The drawing under review shows one solid part. Ordinate dimensions are in mm from its lowest x, y, z. A direction names the side the tool comes from. Coordinates: 2 decimals unless noted, no trailing zeros. Write each loop counter-clockwise with the first axis right and the second up, starting at its lowest first coordinate (ties: lowest second). Pieces come first, ordered by that corner, then holes. Notation, with made-up numbers: (36.25, 67) -> (92.25, 67) arc R24 cw to (92.25, 84) -> close; hole circle Ø4 at (35.25, 63). An arc over 180 degrees is marked (long way). One line per item, written item: value. Start each with the question number.
1) For pin 1 Ø5 at (x, y) = (132, 98.5) entering from +Z, flat-tipped, find the tip position at first contact; note if it passes through.
2) Add section B-B (y = 104.5). State the section outline as (x, z) points, and give its area (3 significant figures).
3) Add section A-A (x = 173.5). State the section outline as (y, z) points, and give its area (3 significant figures).
4) For probe 1 along Z at (x, y) = (302.5, 147.5); probe 2 along Y at (x, z) = (127, 7.25), list the stretches that pass through material, from the lowest coordinate up. Write a range as from..to.
5) Machinability: for the marked faces 1 and 2, which of the approach directions +Z, -Z, +X, -X, +Y, -Y give a long, thin tool a straight path to every point of the face, cutting with its end or side? Answer none if there is none.
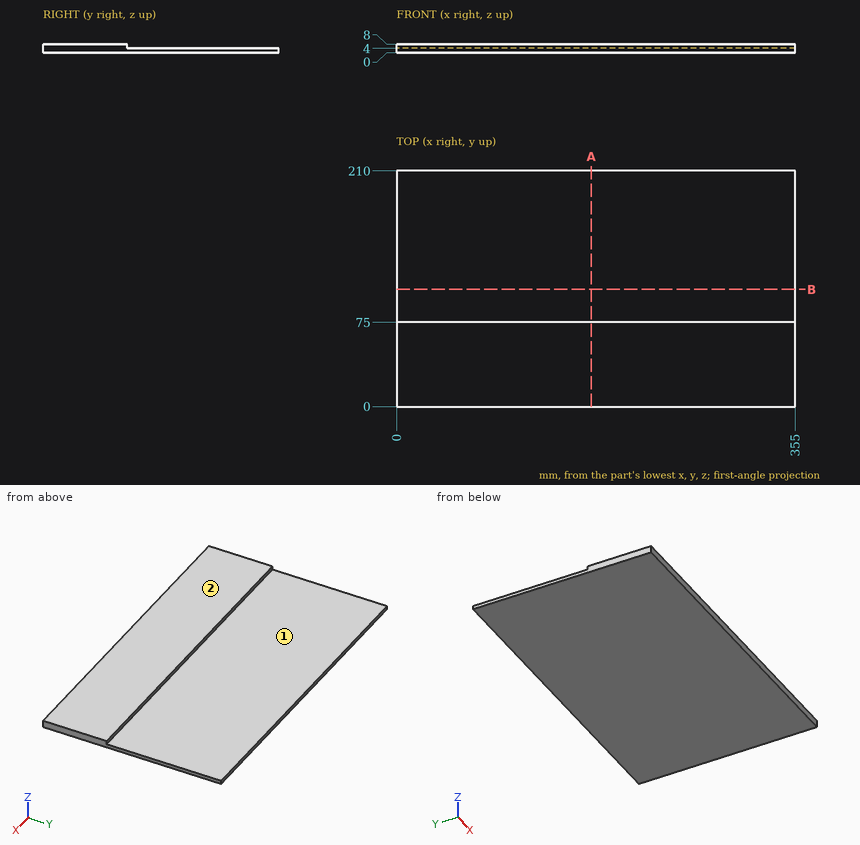
Numbers:
1. pin 1: z = 4
2. outline: (0, 0) -> (355, 0) -> (355, 4) -> (0, 4) -> close
2. area: 1,420 mm²
3. outline: (0, 0) -> (210, 0) -> (210, 4) -> (75, 4) -> (75, 8) -> (0, 8) -> close
3. area: 1,140 mm²
4. probe 1: 0..4
4. probe 2: 0..75
5. face 1: +Z, +X, -X, +Y
5. face 2: +Z, +X, -X, +Y, -Y
